Check sheet for the modelled part. Datum: model origin and axes. Units: mm. Round coordinates to 2 decimals unless told otherwise and drop trailing zeros. Order: outer loops, then holes, each group sorted by start corner. A loop starts at its lowest first (then second) coordinate and runs counter-clockwise, first axis right, second up. Notation, with made-up numbers: M -7,37 L 37,37 A28 cw 37,75 Z; hole C 53,-3.5 d7. An arc over 180 degrees is marked long. One line per item, written item: value. Start each with the question number.
(1) Cross-section at C-C, the plane x = 73. Enter the section's corners in (y, z), and give its area (3 significant figures).
(2) Cross-section at D-D, the plane z = 1.25. Enter the section's corners in (x, y).
(3) Cross-section at B-B, the plane y = 42. Enter the section's corners in (x, z).
(4) Cross-section at A-A, the plane x = 29.5. Enter the section's corners in (y, z), and give its area (3 significant figures).
(5) Depth check by flat-ended pin: pin 1 Ø3 at (x, z) = (63.5, -2.5) entering from -Y; pin 2 Ø1.5 at (y, z) = (39.5, -1.5) entering from +X; pin 3 Ø22 at (x, y) = (60.5, 49.5) entering from -Z; pin 4 Ø0.9 at (x, z) = (25, 1) entering from +Y. Enter the tip coordinate at first touch or a pass-through.
(6) Thickness scan on L1, parallel to Y at x = 73, z = 2.25; L2, parallel to X at y = 31, z = 1.5; L3, parallel to X at y = 48.5, z = 0.5. Record the ranges inside material, lowest first.
from build123d import *

# Parameters (mm, degrees)
F1_DEPTH = 3
F2_W     = 20.5
F2_H     = 12.6
F2_R     = 2
F2_W_2   = 85.5
F2_H_2   = 45.5
F3_DEPTH = 3
F4_W     = 55
F4_H     = 5
F5_DEPTH = 4


with BuildPart() as f1:
    # F0 (on Top) → F1 (new body)
    with BuildSketch(Plane.XY):
        with BuildLine():
            Line((0, 0), (2.5, 0))
            Line((2.5, 0), (143.5, 0))
            Line((143.5, 0), (146, 0))
            Line((146, 0), (146, 4.25))
            Line((146, 4.25), (146, 47))
            ThreePointArc((146, 47), (138.091883, 66.091883), (119, 74))
            Line((119, 74), (27, 74))
            ThreePointArc((27, 74), (7.908117, 66.091883), (0, 47))
            Line((0, 47), (0, 4.25))
            Line((0, 4.25), (0, 0))
        make_face()
    extrude(amount=F1_DEPTH)

    # F2 (on face) → F3 (cut)
    with BuildSketch(Plane.XY.offset(3)):
        with Locations((25.25, 46.3)):
            Rectangle(F2_W, F2_H)
        with Locations((73, 66.5)):
            Circle(F2_R)
        with Locations((90.75, 34.25)):
            Rectangle(F2_W_2, F2_H_2)
    extrude(amount=-F3_DEPTH, mode=Mode.SUBTRACT)

    # F4 (on face) → F5 (join)
    with BuildSketch(Plane(origin=(0, 0, 0), x_dir=(1, 0, 0), z_dir=(0, 0, -1))):
        with Locations((52.5, -7)):
            Rectangle(F4_W, F4_H)
    extrude(amount=F5_DEPTH)


solid = f1.part
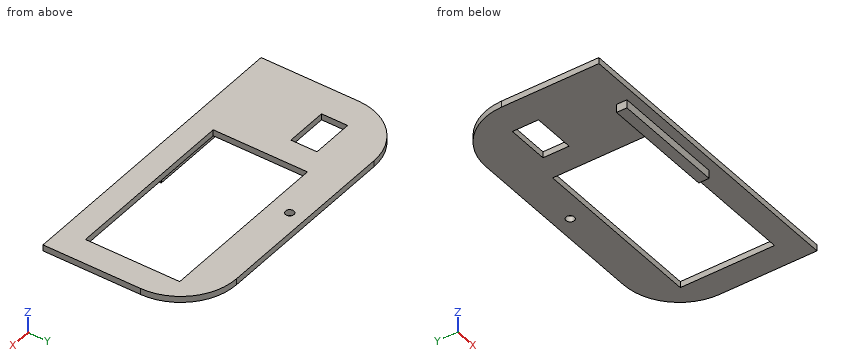
Values found:
1. outline: M 0,0 L 4.5,0 L 4.5,-4 L 9.5,-4 L 9.5,0 L 11.5,0 L 11.5,3 L 0,3 Z; M 57,0 L 64.5,0 L 64.5,3 L 57,3 Z; M 68.5,0 L 74,0 L 74,3 L 68.5,3 Z
1. area: 93.5 mm^2
2. outline: M 0,0 L 146,0 L 146,47 A27 ccw 119,74 L 27,74 A27 ccw 0,47 Z; hole M 15,40 L 35.5,40 L 35.5,52.6 L 15,52.6 Z; hole M 48,11.5 L 133.5,11.5 L 133.5,57 L 48,57 Z; hole C 73,66.5 d4
3. outline: M 0,0 L 15,0 L 15,3 L 0,3 Z; M 35.5,0 L 48,0 L 48,3 L 35.5,3 Z; M 133.5,0 L 146,0 L 146,3 L 133.5,3 Z
4. outline: M 0,0 L 4.5,0 L 4.5,-4 L 9.5,-4 L 9.5,0 L 40,0 L 40,3 L 0,3 Z; M 52.6,0 L 74,0 L 74,3 L 52.6,3 Z
4. area: 204 mm^2
5. pin 1: y = 4.5
5. pin 2: through
5. pin 3: z = 0
5. pin 4: y = 73.96
6. L1: 0 to 11.5, 57 to 64.5, 68.5 to 74
6. L2: 0 to 48, 133.5 to 146
6. L3: 0.04 to 15, 35.5 to 48, 133.5 to 145.96
